```python
from build123d import *

# Parameters (mm, degrees)
SKETCH1_R           = 19.05
SKETCH1_R_2         = 3.175
BOSS_EXTRUDE1_DEPTH = 6.35
BOSS_EXTRUDE3_DEPTH = 6.35
CIRPATTERN2_DEPTH   = 6.35
SKETCH4_R           = 1.5875
BOSS_EXTRUDE4_DEPTH = 6.35


# Read off the part's stored shape, not the designer's step: CirPattern2
with BuildPart() as part:
    # Sketch1 → Boss-Extrude1 (new body)
    with BuildSketch(Plane(origin=(0, 0, 0), x_dir=(1, 0, 0), z_dir=(0, 1, 0))):
        with Locations(Location((0, 0, 0), (0, 0, 270))):
            Circle(SKETCH1_R)
        with Locations(Location((0, 0, 0), (0, 0, 270))):
            Circle(SKETCH1_R_2, mode=Mode.SUBTRACT)
    extrude(amount=BOSS_EXTRUDE1_DEPTH)

    # Sketch3 → Boss-Extrude3 (add)
    with BuildSketch(Plane(origin=(0, 0, 0), x_dir=(1, 0, 0), z_dir=(0, 1, 0))):
        with BuildLine():
            ThreePointArc((-18.32709122, 5.198098444), (-19.680979383, 5.197152008), (-21.013329851, 4.956618665))
            ThreePointArc((-21.013329851, 4.956618665), (-21.175154204, 4.212000052), (-21.310601203, 3.462134657))
            ThreePointArc((-21.310601203, 3.462134657), (-20.171718001, 2.730042376), (-18.921250622, 2.211057413))
            ThreePointArc((-18.921250622, 2.211057413), (-18.683959592, 3.716470634), (-18.32709122, 5.198098444))
        make_face()
    extrude(amount=BOSS_EXTRUDE3_DEPTH)

    # CirPattern2 outline → CirPattern2 (add)
    with BuildSketch(Plane(origin=(0, 0, 0), x_dir=(1, 0, 0), z_dir=(0, 1, 0))):
        with BuildLine():
            ThreePointArc((-17.704260875, 7.032897477), (-17.085425728, 8.425599549), (-16.357243856, 9.764377784))
            ThreePointArc((-16.357243856, 9.764377784), (-17.665244353, 10.113875638), (-19.014450689, 10.226375946))
            ThreePointArc((-19.014450689, 10.226375946), (-19.36348249, 9.549012822), (-19.688393689, 8.859754733))
            ThreePointArc((-19.688393689, 8.859754733), (-18.777796417, 7.857843228), (-17.704260875, 7.032897477))
        make_face()
        with BuildLine():
            ThreePointArc((-15.280755006, 11.375457202), (-14.322548335, 12.560537779), (-13.272677354, 13.665230916))
            ThreePointArc((-13.272677354, 13.665230916), (-14.445652113, 14.341355358), (-15.719768136, 14.799222606))
            ThreePointArc((-15.719768136, 14.799222606), (-16.232221443, 14.235276148), (-16.724454683, 13.653597166))
            ThreePointArc((-16.724454683, 13.653597166), (-16.104199039, 12.450145051), (-15.280755006, 11.375457202))
        make_face()
        with BuildLine():
            ThreePointArc((-11.375457197, -15.280755), (-12.560537774, -14.322548329), (-13.66523091, -13.272677349))
            ThreePointArc((-13.66523091, -13.272677349), (-14.341355358, -14.445652113), (-14.799222606, -15.719768136))
            ThreePointArc((-14.799222606, -15.719768136), (-14.235276148, -16.232221443), (-13.653597166, -16.724454683))
            ThreePointArc((-13.653597166, -16.724454683), (-12.450145051, -16.104199039), (-11.375457197, -15.280755))
        make_face()
        with BuildLine():
            ThreePointArc((-14.942798311, -11.81589093), (-15.839496111, -10.583612937), (-16.634821136, -9.28359982))
            ThreePointArc((-16.634821136, -9.28359982), (-17.59149541, -10.241612555), (-18.363526703, -11.353809363))
            ThreePointArc((-18.363526703, -11.353809363), (-17.95142893, -11.994761331), (-17.516969515, -12.620771728))
            ThreePointArc((-17.516969515, -12.620771728), (-16.193990063, -12.33312711), (-14.942798311, -11.81589093))
        make_face()
        with BuildLine():
            ThreePointArc((-17.491812414, -7.545793421), (-18.039018964, -6.123421813), (-18.470775793, -4.661860306))
            ThreePointArc((-18.470775793, -4.661860306), (-19.642804121, -5.339624026), (-20.676386801, -6.214107244))
            ThreePointArc((-20.676386801, -6.214107244), (-20.444221496, -6.939878056), (-20.18658934, -7.657004037))
            ThreePointArc((-20.18658934, -7.657004037), (-18.834241415, -7.72157295), (-17.491812414, -7.545793421))
        make_face()
        with BuildLine():
            ThreePointArc((-21.580185309, -0.650923987), (-21.543774153, -1.41205356), (-21.480526461, -2.171424174))
            ThreePointArc((-21.480526461, -2.171424174), (-20.190970338, -2.583806354), (-18.84878841, -2.761462559))
            ThreePointArc((-18.84878841, -2.761462559), (-19.009212486, -1.245929612), (-19.047977604, 0.277577285))
            ThreePointArc((-19.047977604, 0.277577285), (-20.355488193, -0.073748943), (-21.580185309, -0.650923987))
        make_face()
    extrude(amount=CIRPATTERN2_DEPTH)

    # Sketch4 → Boss-Extrude4 (add)
    with BuildSketch(Plane(origin=(0, 6.35, 0), x_dir=(1, 0, 0), z_dir=(0, 1, 0))):
        with BuildLine():
            Line((-3.175, 3.175), (3.175, 3.175))
            Line((3.175, 3.175), (3.175, 25.399999902))
            ThreePointArc((3.175, 25.399999902), (0, 28.575), (-3.175, 25.399999902))
            Line((-3.175, 25.399999902), (-3.175, 3.175))
        make_face()
        with Locations(Location((0, 25.4, 0), (0, 0, 270))):
            Circle(SKETCH4_R, mode=Mode.SUBTRACT)
    extrude(amount=-BOSS_EXTRUDE4_DEPTH)


solid = part.part
```
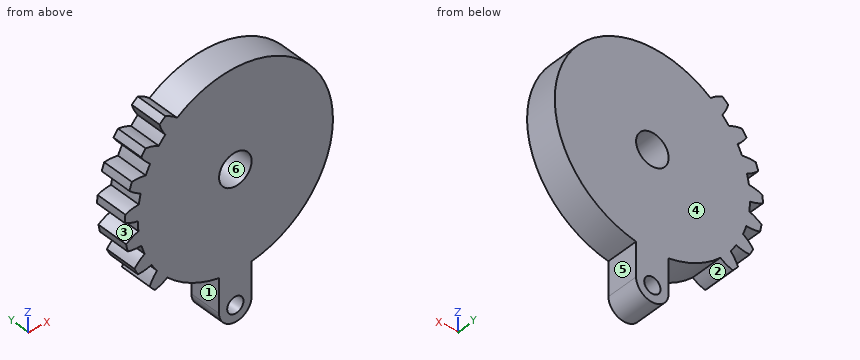
Input: part model. Units: mm. Frame: model coordinates. Face numbers are marked on the shaded views. A direction names the side the tool comes from. Give positions to 0.01 mm unless a question says otherwise; leave off trailing zeros. Order: outer loops, then holes, each group sorted by start corner. A loop starts at its lowest first (then second) coordinate and runs counter-clockwise, first axis right, second up. Notation, with made-up numbers: M 37,76.5 L 81,76.5 A28 ccw 81,107.5 Z; hole C -5,70 d11. An arc over 180 degrees is marked long. One line per question, with ' | ' between items. Start each with the question number.
1. Pull-direction query (X, two-part tool) for the marked faces 4, 5 and 6; classes: released by +X, released by -X, zero draft, split by the parting line, or undercut.
2. First-contact query: pin 1 Ø3 at (x, y) = (-16.5, 2.5) entering from +Z; pin 2 Ø2.5 at (x, z) = (0, -25.4) entering from -Y; pin 3 Ø3 at (x, y) = (9, 4.5) entering from +Z; pin 4 Ø3 at (y, z) = (1.5, -21.5) entering from +X (3 decimals). Flat tips, straight axial feed; report the tip coordinate or a pass-through.
3. Section query C-C (z = -1). Return the cut outline in (x, y), and give its area (3 significant figures).
4. Section query D-D (x = -6). Return the cut outline in (y, z).
5. Section query A-A (x = 0). Count the separate pieces of the cut face and the enclosed holes in it, and give its area (3 significant figures).
6. Material intervals for probe 1 along X at (y, z) = (1, -24.5) (3 decimals); probe 2 along X at (y, z) = (3, -2); probe 3 along X at (y, z) = (2, -19) (3 decimals), sorted ascending. Write a range as [from, to].
7. Access query for the marked faces 1, 2 and 3. Directions: +Z, -Z, +X, -X, +Y, -Y. A direction counts if a zero-diameter tool reaches every point of the face in a straight line with its end or side. Return the directions, or none.
Here are the results:
1) face 4: zero draft | face 5: released by +X | face 6: undercut
2) pin 1: z = 12.62 | pin 2: through | pin 3: z = 17.51 | pin 4: x = 3.175
3) outline: M -19.02,0 L -3.01,0 L -3.01,6.35 L -19.02,6.35 Z; M 3.01,0 L 19.02,0 L 19.02,6.35 L 3.01,6.35 Z | area: 203 mm²
4) outline: M 0,-18.08 L 6.35,-18.08 L 6.35,18.08 L 0,18.08 Z
5) separate pieces: 3 | enclosed holes: 0 | area: 242 mm²
6) probe 1: [-3.175, -1.308], [1.308, 3.175] | probe 2: [-18.94, -2.47], [2.47, 18.94] | probe 3: [-3.175, 3.175]
7) face 1: -Z, -X, +Y, -Y | face 2: -Z, +Y, -Y | face 3: -X, +Y, -Y
